Can you work these out from the drawing? Everything is in mm from the part's minimum corner. A direction names the side the tool comes from. Give positions to 0.01 mm unless a question says otherwise; leave off trailing zeros. Loops run counter-clockwise (first coordinate to the right, second up) from the corner with the lowest first, then second, coordinate; pieces in that order, holes last. Notation, with made-up numbers: (59.25, 42.25) - (66.25, 42.25) arc R24 ccw to (66.25, 70.25) - close; hole circle Ø7 at (73.25, -11.75). An arc over 180 degrees is marked (long way). Answer in a Markdown table with one row per item. Add a question column.
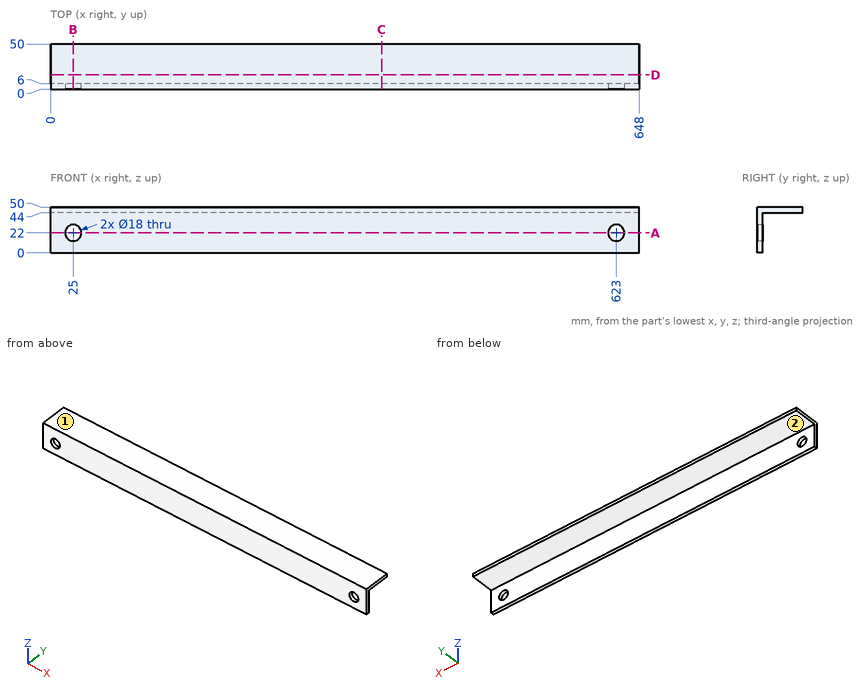
(1) I want a section at D-D on y = 16. Please give me the cut outline in (x, z), then the cut area to 3 significant figures.
(2) For pin 1 Ø22 at (x, z) = (276.5, 18) entering from +Y; pin 2 Ø2 at (x, y) = (500, 16) entering from -Z, each with a flat end and sliding along its axis, tell me the tip position at first contact or that it passes through.
(3) Please list where these lines run through material, in increasing order: line 1 (Z direction, x = 623, y = 3.2); line 2 (Y direction, x = 164, z = 25); line 3 (Z direction, x = 357, y = 46).
(4) I want a section at C-C on x = 364.5. Please give me the cut outline in (y, z), then the cut area to 3 significant figures.
(5) On a 3-axis mill with a long thin cutter (end or side, diameter ignored), from which of +Z, -Z, +X, -X, +Y, -Y can I reach the whole of each face in a straight line? I mean the marked faces 1 and 2. Say none if no direction works.
(6) I want a section at B-B on x = 25. Please give me the cut outline in (y, z).
(7) I want a section at A-A on z = 22. Please give me the cut outline in (x, y).
Reported:
| question | item | result |
|---|---|---|
| 1 | outline | (0, 44) - (648, 44) - (648, 50) - (0, 50) - close |
| 1 | area | 3,890 mm² |
| 2 | pin 1 | y = 6 |
| 2 | pin 2 | z = 44 |
| 3 | line 1 | 0 to 13, 31 to 50 |
| 3 | line 2 | 0 to 6 |
| 3 | line 3 | 44 to 50 |
| 4 | outline | (0, 0) - (6, 0) - (6, 44) - (50, 44) - (50, 50) - (0, 50) - close |
| 4 | area | 564 mm² |
| 5 | face 1 | +Z, +X, -X, +Y, -Y |
| 5 | face 2 | -Z, +X, -X, +Y |
| 6 | outline | (0, 0) - (6, 0) - (6, 13) - (0, 13) - close; (0, 31) - (6, 31) - (6, 44) - (50, 44) - (50, 50) - (0, 50) - close |
| 7 | outline | (0, 0) - (16, 0) - (16, 6) - (0, 6) - close; (34, 0) - (614, 0) - (614, 6) - (34, 6) - close; (632, 0) - (648, 0) - (648, 6) - (632, 6) - close |
